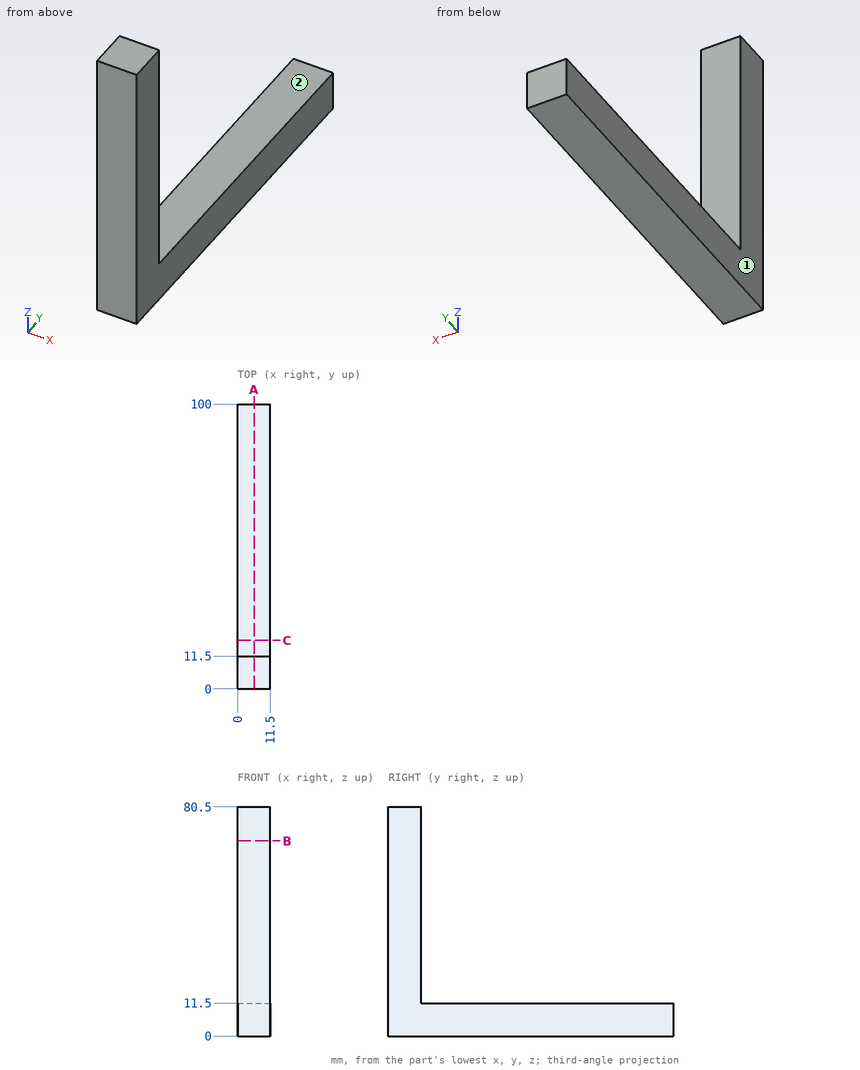
Could you check a few things on this drawing? It's one solid part, dimensions in mm from its lowest x, y, z. A direction names the side the tool comes from. Coordinates: 2 decimals unless noted, no trailing zeros. Order: outer loops, then holes, each group sorted by start corner. A loop starts at its lowest first (then second) coordinate and runs counter-clockwise, first axis right, second up. Notation, with made-up numbers: (43, 16) -> (55, 16) arc R31 ccw to (55, 53) -> close; hole circle Ø6 at (25.5, 3.25). An arc over 180 degrees is marked (long way). One line per item, written item: value. Start each with the question number.
1) If I drill on L1, parallel to Z at x = 2.5, y = 47, over which ranges is the centre line in solid material (lowest first)? Write a range as [from, to].
2) Imagine slicing it at A-A on x = 5.75. List the corners of the cut face in (y, z) for me, plus the area to 3 significant figures.
3) Imagine slicing it at B-B on z = 68.5. List the corners of the cut face in (x, y) for me, plus the area to 3 significant figures.
4) Which directions (+Z, -Z, +X, -X, +Y, -Y) give clear straight access to the entire face, cutting with the end or side of a thin tool? Please do the marked faces 1 and 2.
5) I'm going to push flat-ended pins straight in: pin 1 (2 mm diameter, centred on x = 7.5, z = 71, fed in from -Y); pin 2 (6 mm diameter, centred on x = 3.5, z = 37.5, fed in from +Y). Where does each tip first touch, or does it pass through?
Answer list:
1. L1: z = [0, 11.5]
2. outline: (0, 0) -> (100, 0) -> (100, 11.5) -> (11.5, 11.5) -> (11.5, 80.5) -> (0, 80.5) -> close
2. area: 1,940 mm2
3. outline: (0, 0) -> (11.5, 0) -> (11.5, 11.5) -> (0, 11.5) -> close
3. area: 132 mm2
4. face 1: +Z, -Z, -X, +Y, -Y
4. face 2: +Z, +X, -X, +Y
5. pin 1: stops at y = 0
5. pin 2: stops at y = 11.5
